Read the model definition and answer for the solid it produces. Units are mm, in the model's axes. A direction names the side the tool comes from. Coordinates: 2 decimals unless noted, no trailing zeros. Loops run counter-clockwise (first coordinate to the right, second up) from the corner with the lowest first, then second, coordinate; pieces in that order, holes last. Notation, with made-up numbers: M 13,38 L 48,38 A10 cw 48,48 Z; hole C 7.25,-23.5 d8. An arc over 180 degrees is marked long. Put each result on its own line as item: value.
from build123d import *

# Parameters (mm, degrees)
EXTRUDE_THIN2_DEPTH = 64
RIB1_REACH          = 140.279
SKETCH2_WALL_W      = 394.557408146
SKETCH2_WALL_H      = 2
RIB2_REACH          = 139.364
SKETCH3_WALL_W      = 392.728957338
SKETCH3_WALL_H      = 2
CUT_EXTRUDE1_DEPTH  = 10
RIB9_REACH          = 120.055
SKETCH12_WALL_W     = 298.110143788
SKETCH12_WALL_H     = 1
RIB10_REACH         = 128.685
SKETCH13_WALL_W     = 348.869295694
SKETCH13_WALL_H     = 1
SKETCH14_R          = 2.5
SKETCH14_R_2        = 1.5
BOSS_EXTRUDE1_DEPTH = 15
SKETCH15_W          = 1
SKETCH15_H          = 2.550510257
SKETCH15_W_2        = 2.550510257
SKETCH15_H_2        = 1
BOSS_EXTRUDE2_DEPTH = 10
SKETCH16_R          = 2.5
SKETCH16_R_2        = 1.5
BOSS_EXTRUDE3_DEPTH = 15
SKETCH17_W          = 1
SKETCH17_H          = 2.550510257
SKETCH17_W_2        = 2.550510257
SKETCH17_H_2        = 1
BOSS_EXTRUDE4_DEPTH = 10
SKETCH18_W          = 1
SKETCH18_H          = 2.550510257
SKETCH18_W_2        = 2.550510257
SKETCH18_H_2        = 1
BOSS_EXTRUDE5_DEPTH = 10


with BuildPart() as part:
    # Sketch1 → Extrude-Thin2 (new body)
    with BuildSketch(Plane.XY):
        with BuildLine():
            Line((0, 25), (0, 3))
            ThreePointArc((0, 3), (0.878679656, 0.878679656), (3, 0))
            Line((3, 0), (45, 0))
            Line((45, 0), (117.512360171, 12.568809096))
            ThreePointArc((117.512360171, 12.568809096), (119.295330097, 13.593034489), (120, 15.524733157))
            Line((120, 15.524733157), (120, 25))
            Line((120, 25), (118, 25))
            Line((118, 25), (118, 15.524733157))
            ThreePointArc((118, 15.524733157), (117.765110032, 14.880833601), (117.170786724, 14.539425137))
            Line((117.170786724, 14.539425137), (44.827949394, 2))
            Line((44.827949394, 2), (3, 2))
            ThreePointArc((3, 2), (2.292893219, 2.292893219), (2, 3))
            Line((2, 3), (2, 25))
            Line((2, 25), (0, 25))
        make_face()
    extrude(amount=EXTRUDE_THIN2_DEPTH)

    # Sketch2 wall → Rib1 (add, up to next)
    with BuildSketch(Plane(origin=(60, 25, 0), x_dir=(1, 0, 0), z_dir=(0, 1, 0)), mode=Mode.PRIVATE) as rib1_sk1:
        with Locations((0, -1)):
            Rectangle(SKETCH2_WALL_W, SKETCH2_WALL_H)
    rib1_tool1 = extrude(rib1_sk1.sketch, amount=-RIB1_REACH, mode=Mode.PRIVATE) - part.part
    add(rib1_tool1.solids().sort_by_distance((60, 25, 0))[0])

    # Sketch3 wall → Rib2 (add, up to next)
    with BuildSketch(Plane(origin=(60, 25, 62), x_dir=(1, 0, 0), z_dir=(0, 1, 0)), mode=Mode.PRIVATE) as rib2_sk1:
        with Locations((0, -1)):
            Rectangle(SKETCH3_WALL_W, SKETCH3_WALL_H)
    rib2_tool1 = extrude(rib2_sk1.sketch, amount=-RIB2_REACH, mode=Mode.PRIVATE) - part.part
    add(rib2_tool1.solids().sort_by_distance((60, 25, 62))[0])

    # Sketch8 → Cut-Extrude1 (cut)
    with BuildSketch(Plane(origin=(0.970991275, -5.601872741, 0), x_dir=(0.9853080203996408, 0.17078672353593802, 0), z_dir=(-0.17078672353593802, 0.9853080203996408, 0))):
        with BuildLine():
            Line((72.506630536, -13), (102.506630536, -13))
            ThreePointArc((102.506630536, -13), (107.506630536, -18), (102.506630536, -23))
            Line((102.506630536, -23), (72.506630536, -23))
            ThreePointArc((72.506630536, -23), (67.506630536, -18), (72.506630536, -13))
        make_face()
        with BuildLine():
            Line((72.506630536, -41), (102.506630536, -41))
            ThreePointArc((102.506630536, -41), (107.506630536, -46), (102.506630536, -51))
            Line((102.506630536, -51), (72.506630536, -51))
            ThreePointArc((72.506630536, -51), (67.506630536, -46), (72.506630536, -41))
        make_face()
    extrude(amount=-CUT_EXTRUDE1_DEPTH, mode=Mode.SUBTRACT)

    # Sketch12 wall → Rib9 (add, up to next)
    with BuildSketch(Plane(origin=(24, 25, 32), x_dir=(0, 0, -1), z_dir=(0, 1, 0)), mode=Mode.PRIVATE) as rib9_sk1:
        Rectangle(SKETCH12_WALL_W, SKETCH12_WALL_H)
    rib9_tool1 = extrude(rib9_sk1.sketch, amount=-RIB9_REACH, mode=Mode.PRIVATE) - part.part
    add(rib9_tool1.solids().sort_by_distance((24, 25, 32))[0])

    # Sketch13 wall → Rib10 (add, up to next)
    with BuildSketch(Plane(origin=(71.25, 25, 32), x_dir=(-1, 0, 0), z_dir=(0, 1, 0)), mode=Mode.PRIVATE) as rib10_sk1:
        Rectangle(SKETCH13_WALL_W, SKETCH13_WALL_H)
    rib10_tool1 = extrude(rib10_sk1.sketch, amount=-RIB10_REACH, mode=Mode.PRIVATE) - part.part
    add(rib10_tool1.solids().sort_by_distance((71.25, 25, 32))[0])

    # Sketch14 → Boss-Extrude1 (add)
    with BuildSketch(Plane(origin=(0, 2, 0), x_dir=(1, 0, 0), z_dir=(0, 1, 0))):
        with Locations(Location((15, -32, 0), (0, 0, 270))):
            Circle(SKETCH14_R)
        with Locations(Location((15, -32, 0), (0, 0, 270))):
            Circle(SKETCH14_R_2, mode=Mode.SUBTRACT)
    extrude(amount=BOSS_EXTRUDE1_DEPTH)

    # Sketch15 → Boss-Extrude2 (add)
    with BuildSketch(Plane(origin=(0, 2, 0), x_dir=(1, 0, 0), z_dir=(0, 1, 0))):
        with Locations((15, -28.275255128)):
            Rectangle(SKETCH15_W, SKETCH15_H)
        with Locations((11.275255128, -32)):
            Rectangle(SKETCH15_W_2, SKETCH15_H_2)
        with Locations((15, -35.724744872)):
            Rectangle(SKETCH15_W, SKETCH15_H)
        with Locations((18.724744872, -32)):
            Rectangle(SKETCH15_W_2, SKETCH15_H_2)
    extrude(amount=BOSS_EXTRUDE2_DEPTH)

    # Sketch16 → Boss-Extrude3 (add)
    # profile 1 of 2: a face of its own
    with BuildSketch(Plane(origin=(0.970991275, -5.601872741, 0), x_dir=(0.9853080203996408, 0.17078672353593802, 0), z_dir=(-0.17078672353593802, 0.9853080203996408, 0))):
        with Locations(Location((54.682994606, -18, 0), (0, 0, 180))):
            Circle(SKETCH16_R)
        with Locations(Location((54.682994606, -18, 0), (0, 0, 180))):
            Circle(SKETCH16_R_2, mode=Mode.SUBTRACT)
    # profile 2 of 2: a face of its own
    with BuildSketch(Plane(origin=(0.970991275, -5.601872741, 0), x_dir=(0.9853080203996408, 0.17078672353593802, 0), z_dir=(-0.17078672353593802, 0.9853080203996408, 0))):
        with Locations(Location((54.682994606, -46, 0), (0, 0, 180))):
            Circle(SKETCH16_R)
        with Locations(Location((54.682994606, -46, 0), (0, 0, 180))):
            Circle(SKETCH16_R_2, mode=Mode.SUBTRACT)
    extrude(amount=BOSS_EXTRUDE3_DEPTH)

    # Sketch17 → Boss-Extrude4 (add)
    with BuildSketch(Plane(origin=(0.970991275, -5.601872741, 0), x_dir=(0.9853080203996408, 0.17078672353593802, 0), z_dir=(-0.17078672353593802, 0.9853080203996408, 0))):
        with Locations((54.682994606, -14.275255128)):
            Rectangle(SKETCH17_W, SKETCH17_H)
        with Locations((58.407739478, -18)):
            Rectangle(SKETCH17_W_2, SKETCH17_H_2)
        with Locations((54.682994606, -21.724744872)):
            Rectangle(SKETCH17_W, SKETCH17_H)
        with Locations((50.958249735, -18)):
            Rectangle(SKETCH17_W_2, SKETCH17_H_2)
    extrude(amount=BOSS_EXTRUDE4_DEPTH)

    # Sketch18 → Boss-Extrude5 (add)
    with BuildSketch(Plane(origin=(0.970991275, -5.601872741, 0), x_dir=(0.9853080203996408, 0.17078672353593802, 0), z_dir=(-0.17078672353593802, 0.9853080203996408, 0))):
        with Locations((54.682994606, -42.275255129)):
            Rectangle(SKETCH18_W, SKETCH18_H)
        with Locations((58.407739478, -46)):
            Rectangle(SKETCH18_W_2, SKETCH18_H_2)
        with Locations((54.682994606, -49.724744872)):
            Rectangle(SKETCH18_W, SKETCH18_H)
        with Locations((50.958249735, -46)):
            Rectangle(SKETCH18_W_2, SKETCH18_H_2)
    extrude(amount=BOSS_EXTRUDE5_DEPTH)


solid = part.part
1) Given pin 1 Ø2 at (y, z) = (5.5, 49.5) entering from +X; pin 2 Ø7.5 at (y, z) = (20.5, 23) entering from -X; pin 3 Ø0.9 at (x, z) = (14.5, 32.5) entering from +Y; pin 4 Ø5 at (y, z) = (3, 48) entering from +X, each flat-ended and moving along its own axis, determine where each tip first touches the part or whether it passes through.
Answer list:
pin 1: stops at x = 70.43
pin 2: stops at x = 0
pin 3: stops at y = 2
pin 4: stops at x = 69.96
2) Find section A-A, the plane x = 76. Write down the section's boundary in (y, z).
Answer list:
outline: M 5.37,0 L 25,0 L 25,2 L 7.4,2 L 7.4,13 L 5.37,13 Z; M 5.37,23 L 7.4,23 L 7.4,31.5 L 25,31.5 L 25,32.5 L 7.4,32.5 L 7.4,41 L 5.37,41 Z; M 5.37,51 L 7.4,51 L 7.4,62 L 25,62 L 25,64 L 5.37,64 Z
3) Which of the six approach directions +Z, -Z, +X, -X, +Y, -Y give full straight-line access (tool end or side, diameter ignored) to faces 5 (the flat face through (53.516, 8.509, 49.743)), 6 (the flat face through (88, 8, 23)), 7 (the flat face through (120, 20, 32)), 8 (the flat face through (58, 9, 45.5))?
Answer list:
face 5: none
face 6: +Y, -Y
face 7: +Z, -Z, +X, +Y, -Y
face 8: +Y
4) Find section D-D, the plane z = 5.5. Write down the section's boundary in (x, y).
Answer list:
outline: M 0,3 A3 ccw 3,0 L 45,0 L 117.51,12.57 A3 ccw 120,15.52 L 120,25 L 118,25 L 118,15.52 A1 cw 117.17,14.54 L 44.83,2 L 24.5,2 L 24.5,25 L 23.5,25 L 23.5,2 L 3,2 A1 cw 2,3 L 2,25 L 0,25 Z
5) Find section B-B, the plane y = 23.5. Write down the section's boundary in (x, z), plus the area to 4 significant figures.
Answer list:
outline: M 0,0 L 120,0 L 120,64 L 0,64 Z; hole M 2,2 L 23.5,2 L 23.5,62 L 2,62 Z; hole M 24.5,2 L 118,2 L 118,31.5 L 24.5,31.5 Z; hole M 24.5,32.5 L 118,32.5 L 118,62 L 24.5,62 Z
area: 873.5 mm^2
6) Straight lines are drawn through the part: line 1 (X direction, y = 21.5, z = 59); line 2 (Z direction, x = 48, y = 20); line 3 (X direction, y = 13.25, z = 32). For each, find the intervals that lie inside material, in ascending order. Write a range as [from, to].
Answer list:
line 1: x = [0, 2], [23.5, 24.5], [118, 120]
line 2: z = [0, 2], [31.5, 32.5], [62, 64]
line 3: x = [0, 2], [12.5, 13.5], [16.5, 17.5], [23.5, 118.96]
7) Find section C-C, the plane x = 26. Write down the section's boundary in (y, z), plus the area to 3 significant figures.
Answer list:
outline: M 0,0 L 25,0 L 25,2 L 2,2 L 2,31.5 L 25,31.5 L 25,32.5 L 2,32.5 L 2,62 L 25,62 L 25,64 L 0,64 Z
area: 243 mm^2
8) Determine the mould class of faces 1 (the flat face through (80.749, 6.196, 31.552)), 2 (the flat face through (53.516, 8.509, 14.293)), 3 (the flat face through (54.5, 8.68, 49.74)), 4 (the flat face through (54, 9, 23)) for opening direction Y: released by +Y, released by -Y, zero draft, split by the parting line, or undercut.
Answer list:
face 1: released by -Y
face 2: undercut
face 3: released by +Y
face 4: zero draft
